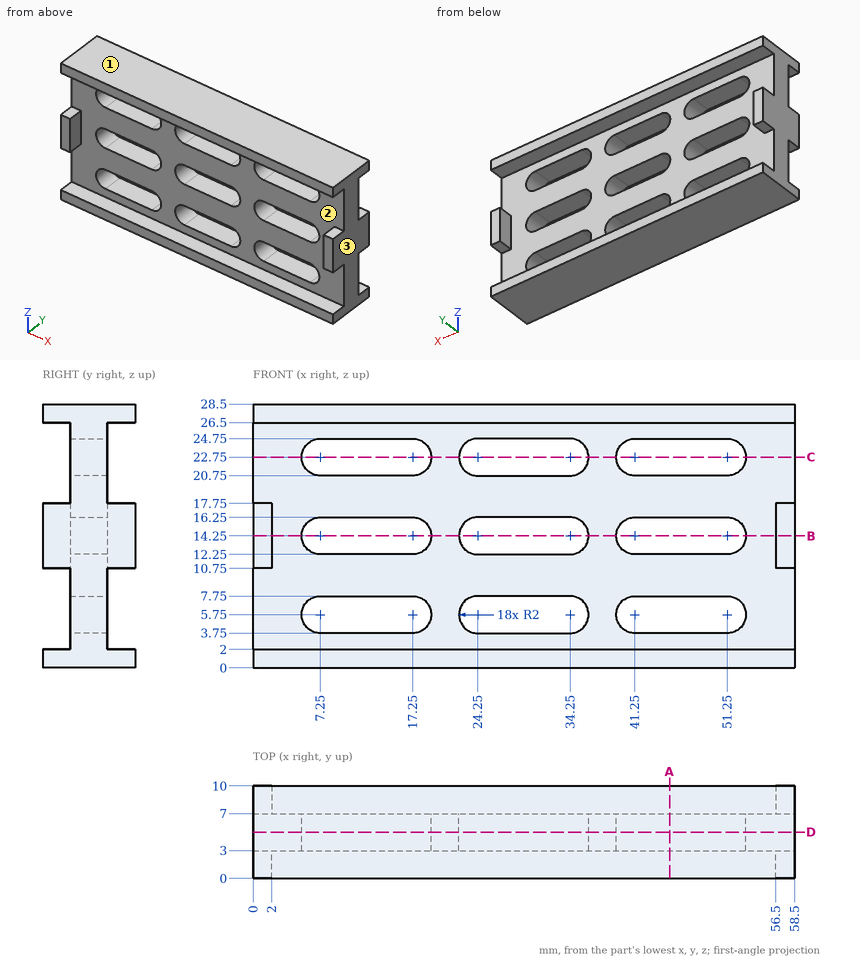
Part print with two shaded views. Sizes in mm from the minimum x, y, z corner. Round coordinates to 2 decimals unless told otherwise and drop trailing zeros. Order: outer loops, then holes, each group sorted by start corner. A loop starts at its lowest first (then second) coordinate and runs counter-clockwise, first axis right, second up. Notation, with made-up numbers: (7, -34) -> (21, -34) arc R25 ccw to (21, 0) -> close; hole circle Ø10 at (57.25, 34). An arc over 180 degrees is marked (long way). Use one line per item in the form item = value.
Item 1: Cut at C-C, the plane z = 22.75. Write the cut outline in (x, y).
Returned:
outline = (0, 3) -> (5.25, 3) -> (5.25, 7) -> (0, 7) -> close; (19.25, 3) -> (22.25, 3) -> (22.25, 7) -> (19.25, 7) -> close; (36.25, 3) -> (39.25, 3) -> (39.25, 7) -> (36.25, 7) -> close; (53.25, 3) -> (58.5, 3) -> (58.5, 7) -> (53.25, 7) -> close
Item 2: Cut at B-B, the plane z = 14.25. Write the cut outline in (x, y).
Returned:
outline = (0, 0) -> (2, 0) -> (2, 3) -> (5.25, 3) -> (5.25, 7) -> (2, 7) -> (2, 10) -> (0, 10) -> close; (19.25, 3) -> (22.25, 3) -> (22.25, 7) -> (19.25, 7) -> close; (36.25, 3) -> (39.25, 3) -> (39.25, 7) -> (36.25, 7) -> close; (53.25, 3) -> (56.5, 3) -> (56.5, 0) -> (58.5, 0) -> (58.5, 10) -> (56.5, 10) -> (56.5, 7) -> (53.25, 7) -> close
Item 3: Flat gauge pins, fed straight in: pin 1 Ø1 at (y, z) = (6, 19) entering from -X; pin 2 Ø10 at (x, z) = (36.5, 10) entering from +Y. Where does each tip first touch, or does it go through?
Returned:
pin_1 = 0
pin_2 = 7
Item 4: Cut at A-A, the plane x = 45. Write the cut outline in (y, z).
Returned:
outline = (0, 0) -> (10, 0) -> (10, 2) -> (7, 2) -> (7, 3.75) -> (3, 3.75) -> (3, 2) -> (0, 2) -> close; (0, 26.5) -> (3, 26.5) -> (3, 24.75) -> (7, 24.75) -> (7, 26.5) -> (10, 26.5) -> (10, 28.5) -> (0, 28.5) -> close; (3, 7.75) -> (7, 7.75) -> (7, 12.25) -> (3, 12.25) -> close; (3, 16.25) -> (7, 16.25) -> (7, 20.75) -> (3, 20.75) -> close
Item 5: Pull direction X, two halves, no side cores. Call the marked faces 1, 2 and 3: released by +X, released by -X, zero draft, split by the parting line, or undercut.
Returned:
face_1 = zero draft
face_2 = undercut
face_3 = released by +X
Item 6: Cut at D-D, the plane y = 5. Give the number of separate pieces and of enclosed holes in the cut face, and give its area (3 significant figures).
Returned:
separate_pieces = 1
enclosed_holes = 9
area = 1,190 mm^2
Item 7: Drill centre lines: line 1 (Z direction, x = 9.5, y = 3.25); line 2 (X direction, y = 4.75, z = 15.75); line 3 (Z direction, x = 26.5, y = 0.5). Where is each one in solid material? Low to high.
Returned:
line_1 = 0 to 3.75, 7.75 to 12.25, 16.25 to 20.75, 24.75 to 28.5
line_2 = 0 to 5.93, 18.57 to 22.93, 35.57 to 39.93, 52.57 to 58.5
line_3 = 0 to 2, 26.5 to 28.5
